from build123d import *

# Parameters (mm, degrees)
SKETCH_1_W                  = 1
SKETCH_1_H                  = 1.9
SKETCH_1_W_2                = 2
SKETCH_1_H_2                = 60
EXTRUDE_1_DEPTH             = 90
SKETCH_2_W                  = 2
SKETCH_2_H                  = 24
CUT_EXTRUDE_1_DEPTH         = 117.034477635
SKETCH_4_W                  = 1
SKETCH_4_H                  = 0.1
EXTRUDE_2_DEPTH             = 3
SKETCH_5_W                  = 2
SKETCH_5_H                  = 24
EXTRUDE_3_DEPTH             = 10
SKETCH_6_W                  = 42
SKETCH_6_H                  = 60
EXTRUDE_4_DEPTH             = 2
EXTRUDE_5_REACH             = 122.702
SKETCH_8_W                  = 10
SKETCH_8_H                  = 2
CUT_EXTRUDE_2_REACH         = 127.571
SKETCH_7_R                  = 5
FILLET_1_R                  = 14
FILLET_2_R                  = 16
FILLET_4_R                  = 8
FILLET_5_R                  = 10
FILLET_6_R                  = 4
FILLET_7_R                  = 6
FILLET_8_R                  = 5
FILLET_9_R                  = 1
EXTRUDE_6_REACH             = 115.723
SKETCH_10_W                 = 1
SKETCH_10_H                 = 1
EXTRUDE_6_DIRECTION_2_DEPTH = 20
SKETCH_11_W                 = 1
SKETCH_11_H                 = 1
EXTRUDE_7_DEPTH             = 50
SKETCH_12_W                 = 33
SKETCH_12_H                 = 1
EXTRUDE_8_DEPTH             = 10
SKETCH_13_W                 = 83
SKETCH_13_H                 = 1
EXTRUDE_9_DEPTH             = 1


with BuildPart() as part:
    # Sketch 1 → Extrude 1 (new body)
    with BuildSketch(Plane(origin=(0, 0, 0), x_dir=(0, 0, -1), z_dir=(1, 0, 0))):
        Polygon((18, 60), (2, 60), (2, 58), (18, 58), (18, 58.1), align=None)
        with Locations((18.5, 59.05)):
            Rectangle(SKETCH_1_W, SKETCH_1_H)
        Polygon((40, 60), (19, 60), (19, 58.1), (19, 58), (40, 58), align=None)
        with Locations((1, 30)):
            Rectangle(SKETCH_1_W_2, SKETCH_1_H_2)
        Polygon((40, 2), (40, 0), (42, 0), (42, 60), (40, 60), (40, 58), align=None)
        Polygon((19, 1.9), (19, 0), (40, 0), (40, 2), (19, 2), align=None)
        with Locations((18.5, 0.95)):
            Rectangle(SKETCH_1_W, SKETCH_1_H)
        Polygon((2, 2), (2, 0), (18, 0), (18, 1.9), (18, 2), align=None)
    extrude(amount=-EXTRUDE_1_DEPTH)

    # Sketch 2 → Cut-Extrude 1 (cut, through all)
    with BuildSketch(Plane(origin=(0, 0, 0), x_dir=(0, 0, -1), z_dir=(1, 0, 0))):
        with Locations((1, 23)):
            Rectangle(SKETCH_2_W, SKETCH_2_H)
    extrude(amount=-CUT_EXTRUDE_1_DEPTH, mode=Mode.SUBTRACT)

    # Sketch 4 → Extrude 2 (add)
    with BuildSketch(Plane.ZY.offset(90)):
        with Locations((-18.5, 58.05)):
            Rectangle(SKETCH_4_W, SKETCH_4_H)
        with Locations((-18.5, 1.95)):
            Rectangle(SKETCH_4_W, SKETCH_4_H)
    extrude(amount=-EXTRUDE_2_DEPTH)

    # Sketch 5 → Extrude 3 (add)
    with BuildSketch(Plane.ZY.offset(90)):
        Polygon((0, 11), (-2, 11), (-2, 2), (-40, 2), (-40, 58), (-2, 58), (-2, 35), (0, 35), (0, 60), (-42, 60), (-42, 0), (0, 0), align=None)
        with Locations((-1, 23)):
            Rectangle(SKETCH_5_W, SKETCH_5_H)
    extrude(amount=EXTRUDE_3_DEPTH)

    # Sketch 6 → Extrude 4 (add)
    with BuildSketch(Plane.ZY.offset(100)):
        with Locations((-21, 30)):
            Rectangle(SKETCH_6_W, SKETCH_6_H)
    extrude(amount=EXTRUDE_4_DEPTH)

    # Sketch 8 → Extrude 5 (add, up to next)
    with BuildSketch(Plane(origin=(0, 11, 0), x_dir=(1, 0, 0), z_dir=(0, 1, 0)), mode=Mode.PRIVATE) as extrude_5_sk1:
        with Locations((-85, 1)):
            Rectangle(SKETCH_8_W, SKETCH_8_H)
    extrude_5_tool1 = extrude(extrude_5_sk1.sketch, amount=EXTRUDE_5_REACH, mode=Mode.PRIVATE) - part.part
    add(extrude_5_tool1.solids().sort_by_distance((-85, 11, -1))[0])

    # Sketch 7 → Cut-Extrude 2 (cut, up to next)
    with BuildSketch(Plane.XY, mode=Mode.PRIVATE) as cut_extrude_2_sk1:
        with Locations((-90, 25)):
            Circle(SKETCH_7_R)
    cut_extrude_2_tool1 = extrude(cut_extrude_2_sk1.sketch, amount=-CUT_EXTRUDE_2_REACH, mode=Mode.PRIVATE) & part.part
    add(cut_extrude_2_tool1.solids().sort_by_distance((-90, 25, 0))[0], mode=Mode.SUBTRACT)

    # Fillet 1
    fillet_1_edges = [part.edges().sort_by_distance(p)[0] for p in [
        (-50, 58, -2),
    ]]
    fillet(fillet_1_edges, radius=FILLET_1_R)

    # Fillet 2
    fillet_2_edges = [part.edges().sort_by_distance(p)[0] for p in [
        (-51, 60, 0),
    ]]
    fillet(fillet_2_edges, radius=FILLET_2_R)

    # Fillet 4
    fillet_4_edges = [part.edges().sort_by_distance(p)[0] for p in [
        (-50, 2, -40),
        (-50, 58, -40),
    ]]
    fillet(fillet_4_edges, radius=FILLET_4_R)

    # Fillet 5
    fillet_5_edges = [part.edges().sort_by_distance(p)[0] for p in [
        (-51, 60, -42),
        (-51, 0, -42),
    ]]
    fillet(fillet_5_edges, radius=FILLET_5_R)

    # Fillet 6
    fillet_6_edges = [part.edges().sort_by_distance(p)[0] for p in [
        (-50, 2, -2),
    ]]
    fillet(fillet_6_edges, radius=FILLET_6_R)

    # Fillet 7
    fillet_7_edges = [part.edges().sort_by_distance(p)[0] for p in [
        (-51, 0, 0),
    ]]
    fillet(fillet_7_edges, radius=FILLET_7_R)

    # Fillet 8
    fillet_8_edges = [part.edges().sort_by_distance(p)[0] for p in [
        (-102, 60, -24),
        (-102, 55.313708499, -4.686291501),
        (-102, 0, -19),
        (-102, 30, -42),
        (-102, 57.071067812, -39.071067812),
        (-102, 2.928932188, -39.071067812),
        (-102, 25, 0),
        (-102, 1.757359313, -1.757359313),
    ]]
    fillet(fillet_8_edges, radius=FILLET_8_R)

    # Fillet 9
    fillet_9_edges = [part.edges().sort_by_distance(p)[0] for p in [
        (-100, 25, -2),
        (-100, 53.899494937, -6.100505063),
        (-100, 30, -40),
        (-100, 58, -24),
        (-100, 55.656854249, -37.656854249),
        (-100, 4.343145751, -37.656854249),
        (-100, 2, -19),
        (-100, 3.171572875, -3.171572875),
    ]]
    fillet(fillet_9_edges, radius=FILLET_9_R)

    # Sketch 10 → Extrude 6 (add, up to next)
    with BuildSketch(Plane(origin=(-87, 0, 0), x_dir=(0, 0, -1), z_dir=(1, 0, 0)), mode=Mode.PRIVATE) as extrude_6_sk1:
        with Locations((17.3, 57.5)):
            Rectangle(SKETCH_10_W, SKETCH_10_H)
    extrude_6_tool1 = extrude(extrude_6_sk1.sketch, amount=-EXTRUDE_6_REACH, mode=Mode.PRIVATE) - part.part
    # Sketch 10 → Extrude 6 (add, up to next)
    with BuildSketch(Plane(origin=(-87, 0, 0), x_dir=(0, 0, -1), z_dir=(1, 0, 0)), mode=Mode.PRIVATE) as extrude_6_sk2:
        with Locations((19.7, 57.5)):
            Rectangle(SKETCH_10_W, SKETCH_10_H)
    extrude_6_tool2 = extrude(extrude_6_sk2.sketch, amount=-EXTRUDE_6_REACH, mode=Mode.PRIVATE) - part.part
    extrude_6_1 = extrude_6_tool1.solids().sort_by_distance((-87, 57.5, -17.3))[0]
    add(extrude_6_1)
    extrude_6_2 = extrude_6_tool2.solids().sort_by_distance((-87, 57.5, -19.7))[0]
    add(extrude_6_2)
    extrude_6 = extrude_6_1 + extrude_6_2  # Extrude 6 as one shape, for the pattern or mirror that repeats it

    # Sketch 10 → Extrude 6 direction 2 (add)
    with BuildSketch(Plane(origin=(-87, 0, 0), x_dir=(0, 0, -1), z_dir=(1, 0, 0))):
        with Locations((17.3, 57.5)):
            Rectangle(SKETCH_10_W, SKETCH_10_H)
        with Locations((19.7, 57.5)):
            Rectangle(SKETCH_10_W, SKETCH_10_H)
    extrude_6_direction_2 = extrude(amount=EXTRUDE_6_DIRECTION_2_DEPTH)

    # Mirror 1: Extrude 6, Extrude 6 direction 2 across plane
    add(extrude_6.mirror(Plane(origin=(0, 30, 0), x_dir=(0, 0, 1), z_dir=(0, -1, 0))))
    add(extrude_6_direction_2.mirror(Plane(origin=(0, 30, 0), x_dir=(0, 0, 1), z_dir=(0, -1, 0))))

    # Sketch 11 → Extrude 7 (add)
    with BuildSketch(Plane(origin=(-67, 0, 0), x_dir=(0, 0, -1), z_dir=(1, 0, 0))):
        with Locations((19.7, 2.5)):
            Rectangle(SKETCH_11_W, SKETCH_11_H)
        with Locations((17.3, 2.5)):
            Rectangle(SKETCH_11_W, SKETCH_11_H)
    extrude(amount=EXTRUDE_7_DEPTH)

    # Sketch 12 → Extrude 8 (add)
    with BuildSketch(Plane.XZ.offset(-57)):
        with Locations((-83.5, -17.3)):
            Rectangle(SKETCH_12_W, SKETCH_12_H)
        with Locations((-83.5, -19.7)):
            Rectangle(SKETCH_12_W, SKETCH_12_H)
    extrude(amount=EXTRUDE_8_DEPTH)

    # Sketch 13 → Extrude 9 (add)
    with BuildSketch(Plane(origin=(0, 3, 0), x_dir=(1, 0, 0), z_dir=(0, 1, 0))):
        with Locations((-58.5, 19.7)):
            Rectangle(SKETCH_13_W, SKETCH_13_H)
        with Locations((-58.5, 17.3)):
            Rectangle(SKETCH_13_W, SKETCH_13_H)
    extrude(amount=EXTRUDE_9_DEPTH)


solid = part.part
Model file for the job. Use its own axes, mm. A direction names the side the tool comes from. Give positions to 0.01 mm unless a question says otherwise; leave off trailing zeros. Loops run counter-clockwise (first coordinate to the right, second up) from the corner with the lowest first, then second, coordinate; pieces in that order, holes last. Notation, with made-up numbers: (1, 87) -> (25, 87) arc R20 cw to (25, 96) -> close; hole circle Ø8 at (65.25, 61). An arc over 180 degrees is marked (long way). Use a Markdown table: item, result. Add a question column.
(1) Slice it at A-A on y = 25. List the corners of the cut face in (x, z), and give its area (3 significant figures).
(2) Slice it at B-B on x = -14. List the corners of the cut face in (y, z), and give its area (3 significant figures).
(3) Wall check: line 1 along Y through (x, z) = (-56, -30.5); line 2 along X through (y, z) = (22.5, -13.5); line 3 along Z through (x, y) = (-71.5, 32). Give the ranges that are in metal, low to high.
(4) Mould opens along Z. For faces 4 (the flat face through (-48, 60, -24)), 5 (the flat face through (-49, 30, -40)), 6 (the cylindrical face through (-47.821, 55.189, -4.563)) say: +Z half, -Z half, draft (parallel to the pull), parting line (faces both ways), or undercut.
(5) Drop flat-ended pins along their axis: pin 1 Ø10 at (x, y) = (-80, 53) entering from +Z; pin 2 Ø1.6 at (x, y) = (-67.5, 3) entering from -Z; pin 3 Ø18 at (y, z) = (42, -18.5) entering from +X. Give the stop position or say it passes through.
(6) Tool access for faces 1 (the flat face through (-39, 11, -1)), 2 (the cylindrical face through (-50.193, 4.281, -37.594)), 3 (the cylindrical face through (-100, 30, -41)): list every direction of +Z, -Z, +X, -X, +Y, -Y with a clear straight run to the whole face (end or side of a thin tool).
Filled sheet:
| question | item | result |
|---|---|---|
| 1 | outline | (-102, -37) arc R5 ccw to (-97, -42) -> (0, -42) -> (0, -40) -> (-99, -40) arc R1 cw to (-100, -39) -> (-100, -3) arc R1 cw to (-99, -2) -> (-95, -2) -> (-95, 0) -> (-97, 0) arc R5 ccw to (-102, -5) -> close; (-85, -2) -> (-80, -2) -> (-80, 0) -> (-85, 0) -> close |
| 1 | area | 294 mm2 |
| 2 | outline | (0, -32) arc R10 ccw to (10, -42) -> (50, -42) arc R10 ccw to (60, -32) -> (60, -16) arc R16 ccw to (44, 0) -> (35, 0) -> (35, -2) -> (44, -2) arc R14 cw to (58, -16) -> (58, -18) -> (58.1, -18) -> (58.1, -19) -> (58, -19) -> (58, -32) arc R8 cw to (50, -40) -> (10, -40) arc R8 cw to (2, -32) -> (2, -19) -> (1.9, -19) -> (1.9, -18) -> (2, -18) -> (2, -6) arc R4 cw to (6, -2) -> (11, -2) -> (11, 0) -> (6, 0) arc R6 ccw to (0, -6) -> close |
| 2 | area | 311 mm2 |
| 3 | line 1 | 0 to 2, 58 to 60 |
| 3 | line 2 | -102 to -100 |
| 3 | line 3 | -42 to -40 |
| 4 | face 4 | draft |
| 4 | face 5 | undercut |
| 4 | face 6 | +Z half |
| 5 | pin 1 | z = -0.51 |
| 5 | pin 2 | z = -39.85 |
| 5 | pin 3 | x = -67 |
| 6 | face 1 | +Z, +X |
| 6 | face 2 | +X |
| 6 | face 3 | -Z, -X, +Y, -Y |
